from build123d import *

# Parameters (mm, degrees)
F1_DEPTH = 25
F2_R     = 1.5
F3_DEPTH = 25
F4_R     = 1.5
F5_DEPTH = 25
F6_R     = 3.313414


with BuildPart() as f1:
    # F0 (on Front) → F1 (new body)
    with BuildSketch(Plane.XZ):
        with BuildLine():
            Line((-30, -29.771222), (30, -29.771222))
            Line((30, -29.771222), (30, -19.771222))
            Line((30, -19.771222), (15.039818, -19.771222))
            ThreePointArc((15.039818, -19.771222), (16.48651, -7.699644), (9.500786, 2.251013))
            Line((9.500786, 2.251013), (9.500786, 13.742813))
            Line((9.500786, 13.742813), (3, 13.742813))
            Line((3, 13.742813), (3, 4.886871))
            Line((3, 4.886871), (3, -0.22738))
            ThreePointArc((3, -0.22738), (0, -23.84633), (-3, -0.22738))
            Line((-3, -0.22738), (-3, 4.886871))
            Line((-3, 4.886871), (-3, 13.742813))
            Line((-3, 13.742813), (-9.500786, 13.742813))
            Line((-9.500786, 13.742813), (-9.500786, 2.251013))
            ThreePointArc((-9.500786, 2.251013), (-16.48651, -7.699644), (-15.039818, -19.771222))
            Line((-15.039818, -19.771222), (-30, -19.771222))
            Line((-30, -19.771222), (-30, -29.771222))
        make_face()
    extrude(amount=F1_DEPTH)

    # F2 (on face) → F3 (cut)
    with BuildSketch(Plane.XY.offset(-19.771222)):
        with Locations((-23.107162, -12.5)):
            Circle(F2_R)
        with Locations((23.107162, -12.5)):
            Circle(F2_R)
    extrude(amount=-F3_DEPTH, mode=Mode.SUBTRACT)

    # F4 (on face) → F5 (cut)
    with BuildSketch(Plane.YZ.offset(9.500786)):
        with Locations((-18.75, 7.996913)):
            Circle(F4_R)
        with Locations((-6.25, 7.996913)):
            Circle(F4_R)
    extrude(amount=-F5_DEPTH, mode=Mode.SUBTRACT)

    # F6
    f6_edges = [f1.edges().sort_by_distance(p)[0] for p in [
        (-6.250393, -25, 13.742813),
        (6.250393, -25, 13.742813),
        (-6.250393, 0, 13.742813),
        (6.250393, 0, 13.742813),
        (30, -25, -24.771222),
        (30, 0, -24.771222),
        (-30, 0, -24.771222),
        (-30, -25, -24.771222),
        (15.039818, -12.5, -19.771222),
        (-15.039818, -12.5, -19.771222),
    ]]
    fillet(f6_edges, radius=F6_R)


solid = f1.part
Design review of the part built by this model. Coordinates are the model's own, in mm. A direction names the side the tool comes from. Coordinates: 2 decimals unless noted, no trailing zeros. Loops run counter-clockwise (first coordinate to the right, second up) from the corner with the lowest first, then second, coordinate; pieces in that order, holes last.
Item 1: Add section A-A (y = -18.75). Write out the cut boundary in (x, z).
Completed:
outline: (-30, -29.77) - (30, -29.77) - (30, -19.77) - (19.78, -19.77) arc R3.31 cw to (16.56, -15.71) arc R17 ccw to (9.5, 2.25) - (9.5, 6.5) - (3, 6.5) - (3, -0.23) arc R12 cw (long way) to (-3, -0.23) - (-3, 6.5) - (-9.5, 6.5) - (-9.5, 2.25) arc R17 ccw to (-16.56, -15.71) arc R3.31 cw to (-19.78, -19.77) - (-30, -19.77) - close; (-9.5, 9.5) - (-3, 9.5) - (-3, 13.74) - (-9.5, 13.74) - close; (3, 9.5) - (9.5, 9.5) - (9.5, 13.74) - (3, 13.74) - close
Item 2: Add section D-D (y = -12.5). Write out the cut boundary in (x, z), and give its area (3 significant figures).
Completed:
outline: (-30, -29.77) - (-24.61, -29.77) - (-24.61, -19.77) - (-30, -19.77) - close; (-21.61, -29.77) - (21.61, -29.77) - (21.61, -19.77) - (19.78, -19.77) arc R3.31 cw to (16.56, -15.71) arc R17 ccw to (9.5, 2.25) - (9.5, 13.74) - (3, 13.74) - (3, -0.23) arc R12 cw (long way) to (-3, -0.23) - (-3, 13.74) - (-9.5, 13.74) - (-9.5, 2.25) arc R17 ccw to (-16.56, -15.71) arc R3.31 cw to (-19.78, -19.77) - (-21.61, -19.77) - close; (24.61, -29.77) - (30, -29.77) - (30, -19.77) - (24.61, -19.77) - close
area: 909 mm2
Item 3: Wall thickness on L1, parallel to X at y = -6.5, z = 6; L2, parallel to Z at x = 7, y = -6.25; L3, parallel to Z at x = 6.5, y = -18.75: over which ranges is each line inside the solid? List them lowest first.
Completed:
L1: x = -9.5 to -3, 3 to 9.5
L2: z = -29.77 to -21.59, -2.1 to 6.5, 9.5 to 13.74
L3: z = -29.77 to -21.93, -1.76 to 6.5, 9.5 to 13.74
Item 4: For faces 4 (the cylindrical face through (-6.2, -20.25, 8.06)), 5 (the flat face through (3, -12, 7)), 6 (the flat face through (25, -12, -19.771)), list the 3-axis set-ups (+Z, -Z, +X, -X, +Y, -Y) from which the entire face can be reached by the end or side of a thin tool; tool diameter is ignored.
Completed:
face 4: +X, -X
face 5: +Z, +Y, -Y
face 6: +Z, +X, +Y, -Y
Item 5: Draft analysis for pull direction X (two halves, no side actions). For faces 1 (the cylindrical face through (-6.3, -0.9, 12.7)), 2 (the cylindrical face through (-21.676, -12.049, -24.701)), 3 (the flat face through (30, -12, -25)), state which applies: pulls with the +X half, pulls with the -X half, needs draft (parallel to the pull), parting line crosses it, or undercut.
Completed:
face 1: needs draft
face 2: undercut
face 3: pulls with the +X half
Item 6: Add section C-C (x = 0). Write out the cut boundary in (y, z).
Completed:
outline: (-25, -29.77) - (0, -29.77) - (0, -23.85) - (-25, -23.85) - close
Item 7: Add section B-B (y = -16). Write out the cut boundary in (x, z).
Completed:
outline: (-30, -29.77) - (30, -29.77) - (30, -19.77) - (19.78, -19.77) arc R3.31 cw to (16.56, -15.71) arc R17 ccw to (9.5, 2.25) - (9.5, 13.74) - (3, 13.74) - (3, -0.23) arc R12 cw (long way) to (-3, -0.23) - (-3, 13.74) - (-9.5, 13.74) - (-9.5, 2.25) arc R17 ccw to (-16.56, -15.71) arc R3.31 cw to (-19.78, -19.77) - (-30, -19.77) - close
Item 8: Clearance check with flat-ended pins moving along their axes: pin 1 (5.5 mm diameter, centred on y = -7, z = 6.5, fed in from +X); pin 2 (2 mm diameter, centred on y = -17, z = -12, fed in from +X); pin 3 (4 mm diameter, centred on y = -18.75, z = 8, fed in from -X). State where each tip first meets the part, or that it passes through.
Completed:
pin 1: stops at x = 9.5
pin 2: stops at x = 17
pin 3: stops at x = -9.5
